```python
from build123d import *

# Parameters (mm, degrees)
SKETCH1_R           = 25
BOSS_EXTRUDE1_DEPTH = 7
SKETCH2_R           = 4
BOSS_EXTRUDE3_DEPTH = 25
SKETCH3_R           = 25
BOSS_EXTRUDE4_DEPTH = 53
SKETCH4_R           = 7
BOSS_EXTRUDE5_DEPTH = 4


with BuildPart() as part:
    # Sketch1 → Boss-Extrude1 (new body)
    with BuildSketch(Plane.XY):
        Circle(SKETCH1_R)
    extrude(amount=BOSS_EXTRUDE1_DEPTH)

    # Sketch2 → Boss-Extrude3 (add)
    with BuildSketch(Plane(origin=(0, 0, 0), x_dir=(-1, 0, 0), z_dir=(0, 0, -1))):
        Circle(SKETCH2_R)
    extrude(amount=BOSS_EXTRUDE3_DEPTH)

    # Sketch3 → Boss-Extrude4 (add)
    with BuildSketch(Plane.XY.offset(7)):
        Circle(SKETCH3_R)
    extrude(amount=BOSS_EXTRUDE4_DEPTH)

    # Sketch4 → Boss-Extrude5 (add)
    with BuildSketch(Plane.XY.offset(60)):
        Circle(SKETCH4_R)
    extrude(amount=BOSS_EXTRUDE5_DEPTH)


solid = part.part
```
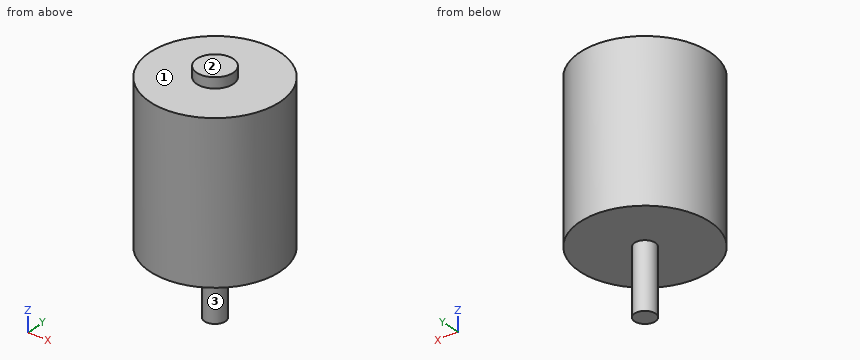
Model file for the job. Use its own axes, mm. Face numbers are marked on the shaded views. A direction names the side the tool comes from. Round coordinates to 2 decimals unless told otherwise and drop trailing zeros. Loops run counter-clockwise (first coordinate to the right, second up) from the corner with the lowest first, then second, coordinate; pieces in that order, holes last. Notation, with made-up numbers: M 19,76 L 64,76 A21 cw 64,88 Z; hole C -29,-10 d8. An arc over 180 degrees is marked long. Put each result on its own line as item: value. Start each with the question number.
Item 1: Drill centre lines: line 1 along Z through (x, y) = (17.5, 2.5); line 2 along Y through (x, z) = (1, 31); line 3 along Y through (x, z) = (0, -12). Where is each one in solid material? Low to high.
Item 2: Cut at D-D (x = -6). List the corners of the cut face in (y, z).
Item 3: Cut at C-C (z = 9). List the corners of the cut face in (x, y).
Item 4: Cut at A-A (x = 0). List the corners of the cut face in (y, z), then the cut area to 3 significant figures.
Item 5: 3-axis set-ups, long thin cutter, end or side, ignore diameter. For the marked faces 1, 2 and 3: which of +Z, -Z, +X, -X, +Y, -Y reach the whole face in a straight line?
Item 6: Drop flat-ended pins along their axis: P1, Ø1, axis at x = 4, z = 28, coming from the -Y side; P2, Ø10, axis at x = 10, y = 9.5, coming from the -Z side; P3, Ø6, axis at y = -9, z = 52.5, coming from the +X side; P4, Ø25, axis at x = 0.5, y = -7, coming from the -Z side. Give the stop position or say it passes through.
Answer block:
1. line 1: 0 to 60
1. line 2: -24.98 to 24.98
1. line 3: -4 to 4
2. outline: M -24.27,0 L 24.27,0 L 24.27,60 L 3.61,60 L 3.61,64 L -3.61,64 L -3.61,60 L -24.27,60 Z
3. outline: C 0,0 d50
4. outline: M -25,0 L -4,0 L -4,-25 L 4,-25 L 4,0 L 25,0 L 25,60 L 7,60 L 7,64 L -7,64 L -7,60 L -25,60 Z
4. area: 3,260 mm2
5. face 1: +Z
5. face 2: +Z, +X, -X, +Y, -Y
5. face 3: -Z
6. P1: y = -24.75
6. P2: z = 0
6. P3: x = 24.27
6. P4: z = -25
